Source: three-view drawing plus pictorial views. Frame: mm from the lowest corner of the part. A direction names the side the tool comes from. Round coordinates to 2 decimals unless told otherwise and drop trailing zeros. Write each loop counter-clockwise with the first axis right and the second up, starting at its lowest first coordinate (ties: lowest second). Pieces come first, ordered by that corner, then holes. Notation, with made-up numbers: M 89,28 L 145,28 A33 ccw 145,58 Z; hole C 70.25,-10 d5. An arc over 180 degrees is marked long. Answer in a Markdown table with one row per item.
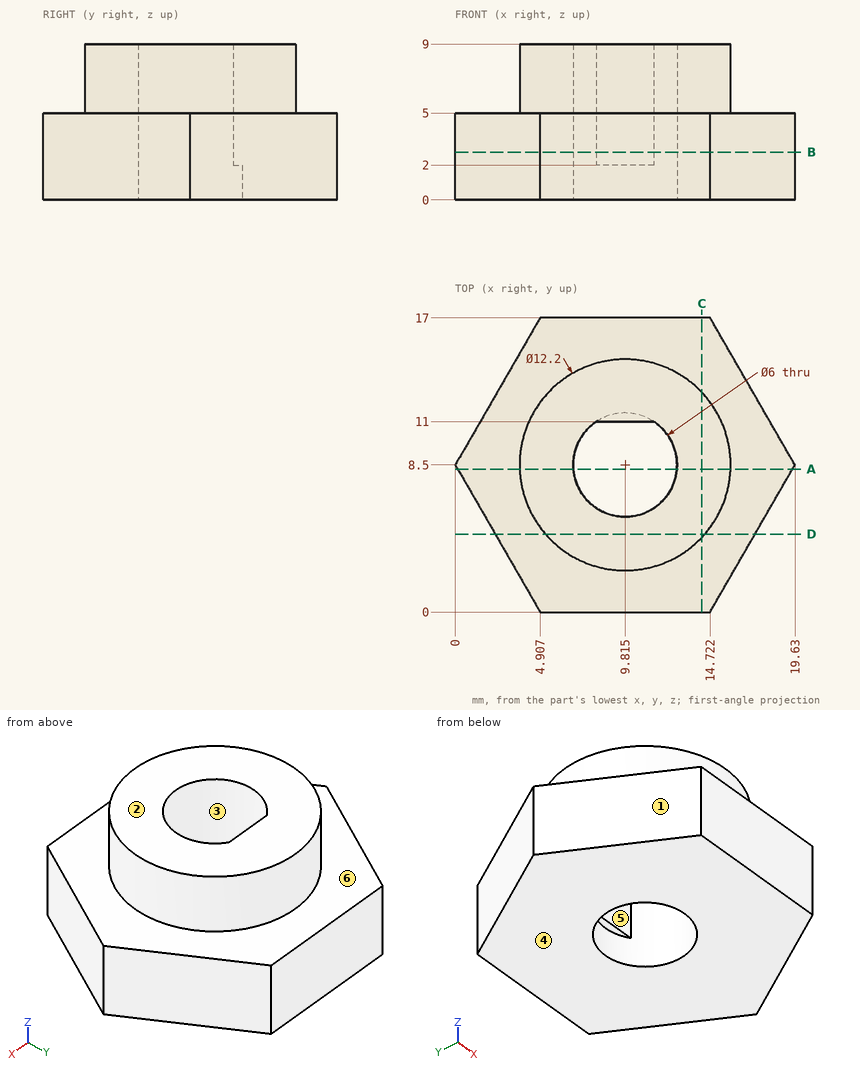
Q1. Contact query for a flat-ended pin moving along its axis: pin 1 Ø5 at (y, z) = (5, 4.5) entering from -X. Output: stop coordinate, or through.
Solutions:
| item | result |
|---|---|
| pin 1 | stops at x = 0.58 |
Q2. Material intervals for probe 1 along Y at (x, z) = (10, 1.5) (1 decimal); probe 2 along Z at (x, y) = (16.75, 3.75); probe 3 along X at (y, z) = (8.25, 2.5) (1 decimal), sorted ascending.
Solutions:
| item | result |
|---|---|
| probe 1 | y = 0 to 5.5, 11.5 to 17 |
| probe 2 | z = 0 to 5 |
| probe 3 | x = 0.1 to 6.8, 12.8 to 19.5 |
Q3. Section D-D (y = 4.5). Return loops of the section in (x, z), and give its area (3 significant figures).
Solutions:
| item | result |
|---|---|
| outline | M 2.31,0 L 17.32,0 L 17.32,5 L 14.42,5 L 14.42,9 L 5.21,9 L 5.21,5 L 2.31,5 Z |
| area | 112 mm2 |
Q4. Pull-direction query (Y, two-part tool) for the marked faces 1, 2 and 3; classes: pulls with the +Y half, pulls with the -Y half, needs draft (parallel to the pull), parting line crosses it, or undercut.
Solutions:
| item | result |
|---|---|
| face 1 | pulls with the -Y half |
| face 2 | needs draft |
| face 3 | undercut |
Q5. Access query for the marked faces 4, 5 and 6. Directions: +Z, -Z, +X, -X, +Y, -Y. A direction counts if a zero-diameter tool reaches every point of the face in a straight line with its end or side. Return the directions, or none.
Solutions:
| item | result |
|---|---|
| face 4 | -Z, +X, -X, +Y, -Y |
| face 5 | +Z, -Z |
| face 6 | +Z |
Q6. Section A-A (y = 8.25). Return loops of the section in (x, z) (1 decimal).
Solutions:
| item | result |
|---|---|
| outline | M 0.1,0 L 6.8,0 L 6.8,9 L 3.7,9 L 3.7,5 L 0.1,5 Z; M 12.8,0 L 19.5,0 L 19.5,5 L 15.9,5 L 15.9,9 L 12.8,9 Z |
Q7. Section B-B (z = 2.75). Return loops of the section in (x, y) (1 decimal).
Solutions:
| item | result |
|---|---|
| outline | M 0,8.5 L 4.9,0 L 14.7,0 L 19.6,8.5 L 14.7,17 L 4.9,17 Z; hole M 8.2,11 A3 ccw long 11.5,11 Z |
Q8. Section C-C (x = 14.25). Return loops of the section in (y, z).
Solutions:
| item | result |
|---|---|
| outline | M 0,0 L 17,0 L 17,5 L 12.69,5 L 12.69,9 L 4.31,9 L 4.31,5 L 0,5 Z |
